Work out the finished part from the listing and answer in its coordinate system (mm). A direction names the side the tool comes from. Round coordinates to 2 decimals unless told otherwise and drop trailing zeros. Write each loop counter-clockwise with the first axis right and the second up, starting at its lowest first coordinate (ties: lowest second). Pieces come first, ordered by that corner, then holes. Notation, with made-up numbers: (-33, 38) - (24, 38) arc R14 cw to (24, 44) - close; hole circle Ø6 at (20, 65). An arc over 180 degrees is marked (long way). Answer as a JSON object with one key per item and string values.
```python
from build123d import *

# Parameters (mm, degrees)
SKETCH1_R           = 70
SKETCH4_R           = 25
CUT_EXTRUDE1_DEPTH  = 50
SKETCH5_R           = 70
BOSS_EXTRUDE2_DEPTH = 70
SKETCH6_R           = 25
BOSS_EXTRUDE3_DEPTH = 50


with BuildPart() as part:
    # Sweep1: sweep along a path in Sketch2
    with BuildLine(Plane(origin=(0, 0, 0), x_dir=(1, 0, 0), z_dir=(0, 1, 0))) as sweep1_path:
        ThreePointArc((70, -70), (49.497474683, -20.502525317), (0, 0))
    # Sketch1 → Sweep1 (sweep)
    with BuildSketch(Plane(origin=(0, 0, 0), x_dir=(0, 0, -1), z_dir=(1, 0, 0))):
        Circle(SKETCH1_R)
    sweep(path=sweep1_path.line)

    # Sketch4 → Cut-Extrude1 (cut)
    with BuildSketch(Plane.ZY):
        Circle(SKETCH4_R)
    extrude(amount=-CUT_EXTRUDE1_DEPTH, mode=Mode.SUBTRACT)

    # Sketch5 → Boss-Extrude2 (add)
    with BuildSketch(Plane.XY.offset(70)):
        with Locations(Location((70, 0, 0), (0, 0, 180))):
            Circle(SKETCH5_R)
    extrude(amount=BOSS_EXTRUDE2_DEPTH)

    # Sketch6 → Boss-Extrude3 (add)
    with BuildSketch(Plane.XY.offset(140)):
        with Locations((70, 0)):
            Circle(SKETCH6_R)
    extrude(amount=BOSS_EXTRUDE3_DEPTH)


solid = part.part
```
Item 1: For faces 1 (the cylindrical face through (45.024, 1.099, 164.65)), 2 (the flat face through (70, 0, 190)), determine the directions among +Z, -Z, +X, -X, +Y, -Y from which every point of the face is accessible in a straight line to the end or side of a thin tool.
Results found:
{"face 1": "+Z", "face 2": "+Z, +X, -X, +Y, -Y"}
Item 2: A cutting plane is placed at A-A (y = 49). Write down the section's boundary in (x, z), and give its area (3 significant figures).
Results found:
{"outline": "(0, -49.99) arc R119.99 ccw to (119.99, 70) - (119.99, 140) - (20.01, 140) - (20.01, 70) arc R20.01 cw to (0, 49.99) - close", "area": "18,000 mm²"}
Item 3: A cutting plane is placed at D-D (y = -40). Write down the section's boundary in (x, z).
Results found:
{"outline": "(0, -57.45) arc R127.45 ccw to (127.45, 70) - (127.45, 140) - (12.55, 140) - (12.55, 70) arc R12.55 cw to (0, 57.45) - close"}
Item 4: A cutting plane is placed at B-B (z = 88). Write down the section's boundary in (x, y), and give its area (3 significant figures).
Results found:
{"outline": "circle Ø140 at (70, 0)", "area": "15,400 mm²"}
Item 5: A cutting plane is placed at C-C (y = 15). Write down the section's boundary in (x, z), and give its area (3 significant figures).
Results found:
{"outline": "(0, -68.37) arc R138.37 ccw to (138.37, 70) - (138.37, 140) - (90, 140) - (90, 190) - (50, 190) - (50, 140) - (1.63, 140) - (1.63, 70) arc R1.63 cw to (0, 68.37) - (0, 20) - (50, 20) - (50, -20) - (0, -20) - close", "area": "24,600 mm²"}
Item 6: Determine the mould class of faces 3 (the flat face through (40, -1, 140)), 4 (the flat face through (50, 0, 0)), 5 (the cylindrical face through (125.55, 42.594, 104.51)), 6 (the cylindrical face through (24.65, 7.509, 23.846)) for opening direction Z: pulls with the +Z half, pulls with the -Z half, needs draft (parallel to the pull), parting line crosses it, or undercut.
Results found:
{"face 3": "pulls with the +Z half", "face 4": "undercut", "face 5": "needs draft", "face 6": "undercut"}
Item 7: Consider line 1 along Y through (x, z) = (20, 0); line 2 along Y through (x, z) = (15, 0); line 3 along X through (y, z) = (-36, 123). Determine where each line is inside the solid, lowest interval first.
Results found:
{"line 1": "-69.94 to -25, 25 to 69.94", "line 2": "-69.98 to -25, 25 to 69.98", "line 3": "9.97 to 130.03"}
Item 8: Each of these flat-tipped pins is pushed along its axis until it touches: P1, Ø3, axis at x = 92, y = 3.5, coming from the -Z side; P2, Ø4, axis at y = -2.5, z = 88, coming from the +X side; P3, Ø2, axis at y = 4.5, z = -36.5, coming from the +X side. Where does it stop, or does it pass through?
Results found:
{"P1": "z = -36.7", "P2": "x = 140", "P3": "x = 91.81"}
